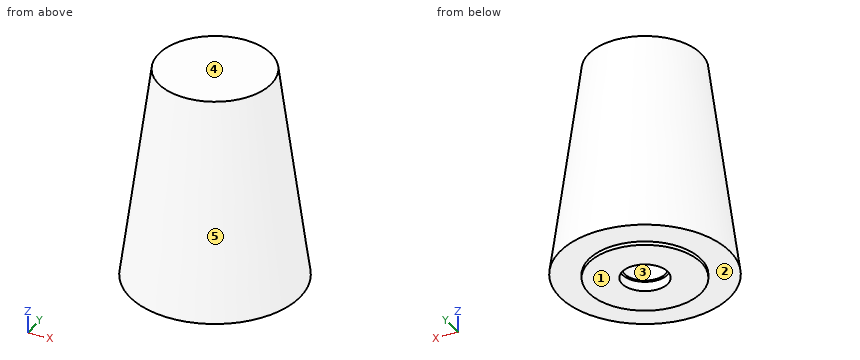
from build123d import *

# Parameters (mm, degrees)
F3_D           = 34.12998
F3_DEPTH       = 55
F3_CBORE_D     = 38.1
F3_CBORE_DEPTH = 8
F3_TIP         = 10.2536804551


with BuildPart() as f1:
    # F0 (on Front) → F1 (revolve)
    with BuildSketch(Plane.XZ):
        Polygon((47, -3), (47, 0), (71, 0), (47, 178), (0, 178), (0, 0), (0, -3), align=None)
    revolve(axis=Axis((0, 0, 89), (0, 0, 1)))

    # F3
    with Locations(Plane(origin=(0, 0, -3), x_dir=(1, 0, 0), z_dir=(0, 0, -1))):
        with Locations((0, 0)):
            CounterBoreHole(F3_D / 2, F3_CBORE_D / 2, F3_CBORE_DEPTH, depth=F3_DEPTH)
            with Locations((0, 0, -(F3_DEPTH + F3_TIP / 2))):  # 118° drill point
                Cone(0, F3_D / 2, F3_TIP, mode=Mode.SUBTRACT)


solid = f1.part
Geometry check sheet. Reference: the model listing, model coordinates, mm. Face numbers are marked on the shaded views. A direction names the side the tool comes from. Give positions to 0.01 mm unless a question says otherwise; leave off trailing zeros. Write each loop counter-clockwise with the first axis right and the second up, starting at its lowest first coordinate (ties: lowest second). Pieces come first, ordered by that corner, then holes. Notation, with made-up numbers: (60, 66.5) - (114, 66.5) arc R12 ccw to (114, 79.5) - close; hole circle Ø11 at (7, 46). An arc over 180 degrees is marked (long way). Put each result on its own line as item: value.
1. Set-up check for the marked faces 1 and 2: record each of +Z, -Z, +X, -X, +Y, -Y from which the full face is reachable in a straight line by a thin tool's end or side.
Ans:
face 1: -Z, +X, -X, +Y, -Y
face 2: -Z
2. Thickness scan on line 1 (Y direction, x = 0, z = 0.5); line 2 (Z direction, x = 7, y = 16); line 3 (Y direction, x = -14, z = 46.5). Record the ranges inside material, lowest first.
Ans:
line 1: y = -70.93 to -19.05, 19.05 to 70.93
line 2: z = 5 to 178
line 3: y = -63.2 to -9.76, 9.76 to 63.2
3. Sectioned sample at C-C, the plane z = 82. Enter the section's corners in (x, y), plus the area to 3 significant figures.
Ans:
outline: circle Ø119.89 at (0, 0)
area: 11,300 mm²
4. Sectioned sample at B-B, the plane z = 10. Enter the section's corners in (x, y) (3 decimals), plus the area to 3 significant figures.
Ans:
outline: circle Ø139.303 at (0, 0); hole circle Ø34.13 at (0, 0)
area: 14,300 mm²
5. Sectioned sample at A-A, the plane z = 158. Enter the section's corners in (x, y), plus the area to 3 significant figures.
Ans:
outline: circle Ø99.39 at (0, 0)
area: 7,760 mm²
6. Go/stop test with flat-tipped pins: pin 1 (5 mm diameter, centred on y = -4.5, z = 41, fed in from +X); pin 2 (5 mm diameter, centred on x = -50, z = 79, fed in from +Y); pin 3 (2 mm diameter, centred on x = -35, z = 113.5, fed in from +Y). Record where each tip stops, or that it passes through.
Ans:
pin 1: stops at x = 65.69
pin 2: stops at y = 37.27
pin 3: stops at y = 44.13
7. Draft check along X on the marked faces 3, 4 and 5. Enter one of: +X half, -X half, draft (parallel to the pull), parting line (faces both ways), or undercut.
Ans:
face 3: undercut
face 4: draft
face 5: parting line
